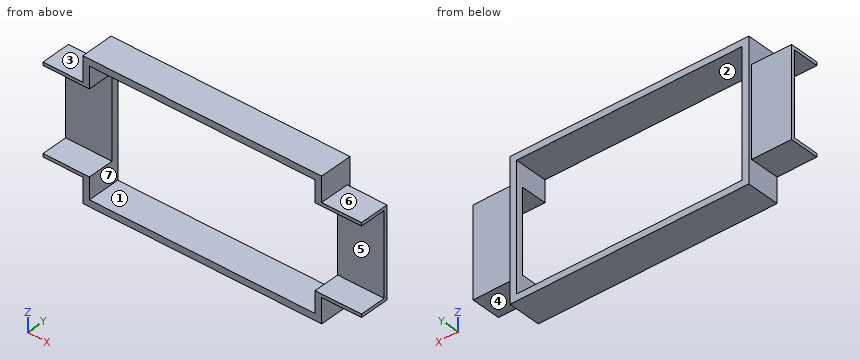
```python
from build123d import *

# Parameters (mm, degrees)
SKETCH_1_W          = 72
SKETCH_1_H          = 42
SKETCH_1_W_2        = 68
SKETCH_1_H_2        = 38
EXTRUDE_1_DEPTH     = 10
SKETCH_2_W          = 25
SKETCH_2_H          = 8
CUT_EXTRUDE_1_DEPTH = 81
EXTRUDE_4_DEPTH     = 12
EXTRUDE_5_DEPTH     = 12


with BuildPart() as part:
    # 草圖1 → 填料-伸長1 (new body)
    with BuildSketch(Plane(origin=(0, 0, 0), x_dir=(1, 0, 0), z_dir=(0, 1, 0))):
        Rectangle(SKETCH_1_W, SKETCH_1_H)
        Rectangle(SKETCH_1_W_2, SKETCH_1_H_2, mode=Mode.SUBTRACT)
    extrude(amount=EXTRUDE_1_DEPTH)

    # 草圖2 → 除料-伸長1 (cut)
    with BuildSketch(Plane(origin=(36, 0, 0), x_dir=(0, 0, -1), z_dir=(1, 0, 0))):
        with Locations((0, 4)):
            Rectangle(SKETCH_2_W, SKETCH_2_H)
    extrude(amount=-CUT_EXTRUDE_1_DEPTH, mode=Mode.SUBTRACT)

    # 草圖7 → 填料-伸長4 (add)
    with BuildSketch(Plane(origin=(36, 0, 0), x_dir=(0, 0, -1), z_dir=(1, 0, 0))):
        Polygon((12.5, 0), (12.5, 8), (-12.5, 8), (-12.5, 0), (-13.5, 0), (-13.5, 9), (13.5, 9), (13.5, 0), align=None)
    extrude(amount=EXTRUDE_4_DEPTH)

    # 草圖9 → 填料-伸長5 (add)
    with BuildSketch(Plane.ZY.offset(36)):
        Polygon((12.5, 8), (12.5, 0), (13.5, 0), (13.5, 9), (-13.5, 9), (-13.5, 0), (-12.5, 0), (-12.5, 8), align=None)
    extrude(amount=EXTRUDE_5_DEPTH)


solid = part.part
```
Geometry check sheet. Reference: the model listing, model coordinates, mm. Face numbers are marked on the shaded views. A direction names the side the tool comes from. Coordinates: 2 decimals unless noted, no trailing zeros. Order: outer loops, then holes, each group sorted by start corner. A loop starts at its lowest first (then second) coordinate and runs counter-clockwise, first axis right, second up. Notation, with made-up numbers: (44, 85) - (91, 85) arc R14 cw to (91, 97) - close; hole circle Ø2 at (44, 46). An arc over 180 degrees is marked (long way). Answer as a JSON object with one key per item and string values. Group by question number.
Item 1: Tool access check on the marked faces 5, 6 and 7. Record the directions out of +Z, -Z, +X, -X, +Y, -Y that give a thin tool (end or side, any length) a straight path to the whole face; none if there is none.
Item 2: Draft check along Z on the marked faces 1, 2, 3 and 4. Enter one of: +Z half, -Z half, draft (parallel to the pull), parting line (faces both ways), or undercut.
Item 3: Scan lines: probe 1 along Z at (x, y) = (-4.5, 3.75); probe 2 along Z at (x, y) = (41, 4.25); probe 3 along X at (y, z) = (1, -13). Record each from-to range of solid material in increasing order.
Item 4: Sectioned sample at D-D, the plane z = -14.5. Record the cut outline in (x, y), and give its area (3 significant figures).
Item 5: Sectioned sample at A-A, the plane x = -2. Record the cut outline in (y, z), and give its area (3 significant figures).
Item 6: Depth check by flat-ended pin: pin 1 Ø4.5 at (x, y) = (41.5, 3.5) entering from -Z; pin 2 Ø9.5 at (x, z) = (-43, -1.5) entering from +Y; pin 3 Ø15.5 at (x, z) = (-40.5, -1.5) entering from -Y; pin 4 Ø5 at (y, z) = (4, -7) entering from +X. Enter the tip coordinate at first touch or a pass-through.
Item 7: Sectioned sample at C-C, the plane y = 3.5. Record the cut outline in (x, z).
Item 8: Sectioned sample at B-B, the plane z = 10. Record the cut outline in (x, y).
Resolved:
{
 "1": {"face 5": "+X, -X, -Y", "face 6": "+Z, +X, +Y, -Y", "face 7": "+Y, -Y"},
 "2": {"face 1": "undercut", "face 2": "undercut", "face 3": "+Z half", "face 4": "-Z half"},
 "3": {"probe 1": "-21 to -19, 19 to 21", "probe 2": "-13.5 to -12.5, 12.5 to 13.5", "probe 3": "-48 to -34, 34 to 48"},
 "4": {"outline": "(-36, 0) - (-34, 0) - (-34, 10) - (-36, 10) - close; (34, 0) - (36, 0) - (36, 10) - (34, 10) - close", "area": "40.0 mm^2"},
 "5": {"outline": "(0, -21) - (10, -21) - (10, -19) - (0, -19) - close; (0, 19) - (10, 19) - (10, 21) - (0, 21) - close", "area": "40.0 mm^2"},
 "6": {"pin 1": "z = -13.5", "pin 2": "y = 9", "pin 3": "y = 8", "pin 4": "through"},
 "7": {"outline": "(-48, -13.5) - (-36, -13.5) - (-36, -21) - (36, -21) - (36, -13.5) - (48, -13.5) - (48, -12.5) - (34, -12.5) - (34, -19) - (-34, -19) - (-34, -12.5) - (-48, -12.5) - close; (-48, 12.5) - (-34, 12.5) - (-34, 19) - (34, 19) - (34, 12.5) - (48, 12.5) - (48, 13.5) - (36, 13.5) - (36, 21) - (-36, 21) - (-36, 13.5) - (-48, 13.5) - close"},
 "8": {"outline": "(-48, 8) - (-34, 8) - (-34, 10) - (-36, 10) - (-36, 9) - (-48, 9) - close; (34, 8) - (48, 8) - (48, 9) - (36, 9) - (36, 10) - (34, 10) - close"}
}
